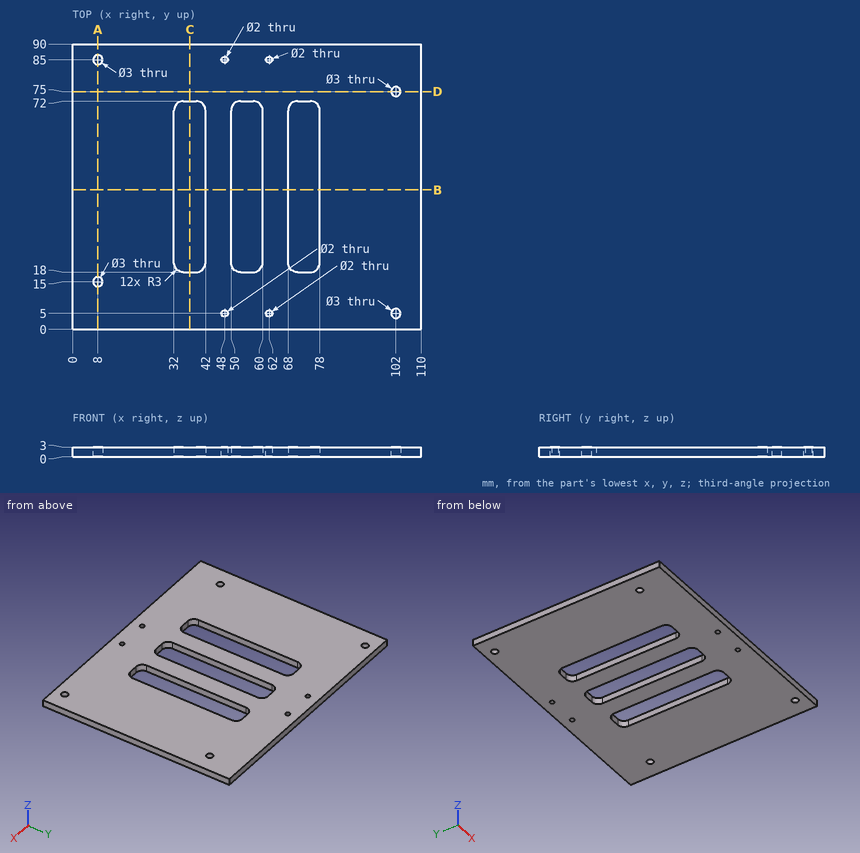
Here's the drawing with two shaded views (mm, measured from the low corner). I have some questions. Give positions to 0.01 mm unless a question says otherwise; leave off trailing zeros. Order: outer loops, then holes, each group sorted by start corner. A loop starts at its lowest first (then second) coordinate and runs counter-clockwise, first axis right, second up. Notation, with made-up numbers: (47.25, 60.5) -> (62.25, 60.5) arc R13 cw to (62.25, 66.5) -> close; hole circle Ø6 at (40, -22). An arc over 180 degrees is marked (long way). Use a Markdown table: item, result. Add a question column.
Item 1: Imagine slicing it at A-A on x = 8. Please give me the cut outline in (y, z), plus the area to 3 significant figures.
Item 2: Imagine slicing it at C-C on x = 37. Please give me the cut outline in (y, z).
Item 3: Imagine slicing it at D-D on y = 75. Please give me the cut outline in (x, z), plus the area to 3 significant figures.
Item 4: Imagine slicing it at B-B on y = 44. Please give me the cut outline in (x, z), plus the area to 3 significant figures.
Item 5: I need wall thicknesses on line 1 (Y direction, x = 8, z = 0.75); line 2 (Y direction, x = 62, z = 0.8); line 3 (X direction, y = 52, z = 2.7). Which ranges of each line are inside material? Lowest first, please.
Data:
| question | item | result |
|---|---|---|
| 1 | outline | (0, 0) -> (13.5, 0) -> (13.5, 3) -> (0, 3) -> close; (16.5, 0) -> (83.5, 0) -> (83.5, 3) -> (16.5, 3) -> close; (86.5, 0) -> (90, 0) -> (90, 3) -> (86.5, 3) -> close |
| 1 | area | 252 mm² |
| 2 | outline | (0, 0) -> (18, 0) -> (18, 3) -> (0, 3) -> close; (72, 0) -> (90, 0) -> (90, 3) -> (72, 3) -> close |
| 3 | outline | (0, 0) -> (100.5, 0) -> (100.5, 3) -> (0, 3) -> close; (103.5, 0) -> (110, 0) -> (110, 3) -> (103.5, 3) -> close |
| 3 | area | 321 mm² |
| 4 | outline | (0, 0) -> (32, 0) -> (32, 3) -> (0, 3) -> close; (42, 0) -> (50, 0) -> (50, 3) -> (42, 3) -> close; (60, 0) -> (68, 0) -> (68, 3) -> (60, 3) -> close; (78, 0) -> (110, 0) -> (110, 3) -> (78, 3) -> close |
| 4 | area | 240 mm² |
| 5 | line 1 | y = 0 to 13.5, 16.5 to 83.5, 86.5 to 90 |
| 5 | line 2 | y = 0 to 4, 6 to 84, 86 to 90 |
| 5 | line 3 | x = 0 to 32, 42 to 50, 60 to 68, 78 to 110 |
